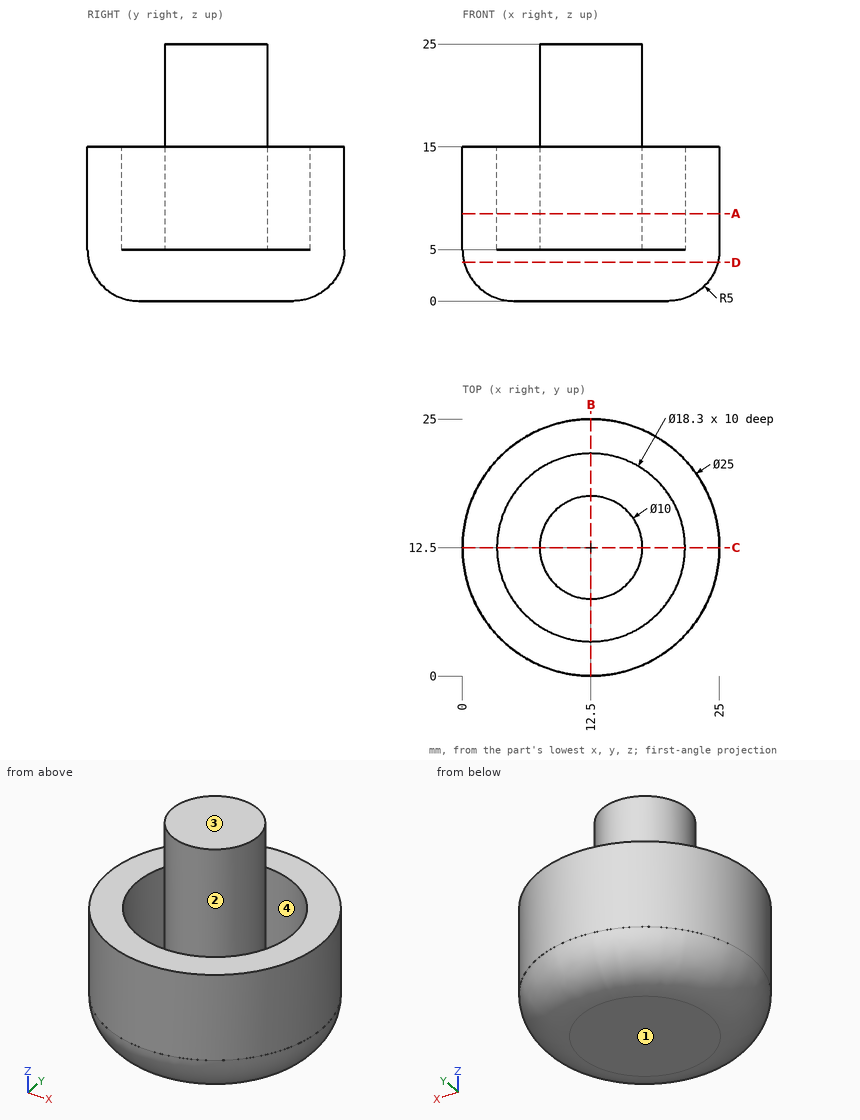
Here's the drawing with two shaded views (mm, measured from the low corner). I have some questions. A direction names the side the tool comes from. Coordinates: 2 decimals unless noted, no trailing zeros. Write each loop counter-clockwise with the first axis right and the second up, starting at its lowest first coordinate (ties: lowest second). Pieces come first, ordered by that corner, then holes.
Item 1: Will these pins go through, and if not, where does the flat tip stop? pin 1 (10 mm diameter, centred on y = 20, z = 22.5, fed in from -X); pin 2 (12 mm diameter, centred on x = 3.5, z = 6, fed in from -Y); pin 3 (1.5 mm diameter, centred on x = 17.5, y = 20.5, fed in from -Z).
Item 2: If we mould it in two halves opening along Y, with no side actions, what happens to the marked faces 3 and 4? For each: +Y half, -Y half, draft (parallel to the pull), parting line (faces both ways), or undercut.
Item 3: I want a section at D-D on z = 3.75. Write out the boundary of the cut face in (x, y).
Item 4: On a 3-axis mill with a long thin cutter (end or side, diameter ignored), from which of +Z, -Z, +X, -X, +Y, -Y can I reach the whole of each face in a straight line? I mean the marked faces 1 and 2. Say none if no direction works.
Item 5: I want a section at A-A on z = 8.5. Write out the boundary of the cut face in (x, y).
Item 6: I want a section at B-B on x = 12.5. Write out the boundary of the cut face in (y, z), and give its area (3 significant figures).
Item 7: If I drill on line 1 (Y direction, x = 12.5, z = 10); line 2 (Y direction, x = 15.5, z = 11) (1 decimal); line 3 (Z direction, x = 6, y = 12.25), over which ranges is the centre line in solid material (lowest first)?
Findings below:
1. pin 1: stops at x = 8.17
1. pin 2: stops at y = 0.37
1. pin 3: stops at z = 0.14
2. face 3: draft
2. face 4: undercut
3. outline: circle Ø24.68 at (12.5, 12.5)
4. face 1: -Z, +X, -X, +Y, -Y
4. face 2: +Z
5. outline: circle Ø25 at (12.5, 12.5); circle Ø10 at (12.5, 12.5); hole circle Ø18.3 at (12.5, 12.5)
6. outline: (0, 5) arc R5 ccw to (5, 0) - (20, 0) arc R5 ccw to (25, 5) - (25, 15) - (21.65, 15) - (21.65, 5) - (17.5, 5) - (17.5, 25) - (7.5, 25) - (7.5, 5) - (3.35, 5) - (3.35, 15) - (0, 15) - close
6. area: 381 mm2
7. line 1: y = 0 to 3.35, 7.5 to 17.5, 21.65 to 25
7. line 2: y = 0.4 to 3.9, 8.5 to 16.5, 21.1 to 24.6
7. line 3: z = 0 to 5
